Source: CAD feature listing. Evaluate the final solid. Frame: model axes, mm. Face numbers are marked on the shaded views. A direction names the side the tool comes from. Give positions to 0.01 mm unless a question says otherwise; leave off trailing zeros. Write each loop counter-clockwise with the first axis right and the second up, starting at its lowest first coordinate (ties: lowest second). Pieces come first, ordered by that corner, then holes. Notation, with made-up numbers: M 21,8 L 30,8 A17 cw 30,21 Z; hole C -1.75,9.25 d5. An arc over 180 degrees is marked long. Use CSV: the item, a comma, the result in double quotes. Start each with the question number.
Autodesk Inventor part; units mm, degrees
ref_plane "YZ Plane" through (0, 0, 0) normal (1, 0, 0) x (0, 1, 0)
ref_plane "XZ Plane" through (0, 0, 0) normal (0, 1, 0) x (-1, 0, 0)
ref_plane "XY Plane" through (0, 0, 0) normal (0, 0, 1) x (1, 0, 0)
sketch "スケッチ1" plane through (0, 0, 0) normal (0, 0, 1) x (1, 0, 0)
  line L0 (-12.5, 3.2) -> (-11.75, 0)
  line L1 (-11.75, 0) -> (11.75, 0)
  line L2 (11.75, 0) -> (12.5, 3.2)
  line L3 (12.5, 3.2) -> (19.5, 3.2)
  line L4 (19.5, 3.2) -> (19.5, -4)
  line L5 (19.5, -4) -> (-19.5, -4)
  line L6 (-19.5, -4) -> (-19.5, 3.2)
  line L7 (-19.5, 3.2) -> (-12.5, 3.2)
  circle A0 centre (0, -21) radius 12.7 construction
  line L8 (-5.5, -4) -> (5.5, -4) construction
  line L9 (5.5, -4) -> (5.5, -7.5) construction
  line L10 (5.5, -7.5) -> (-5.5, -7.5) construction
  line L11 (-5.5, -7.5) -> (-5.5, -4) construction
  circle A1 centre (0, -21) radius 14.7 construction
  line L12 (-19.5, -21) -> (19.5, -21) construction
  line L13 (-18.75, -24.8) -> (-13.25, -24.8) construction
  line L14 (-13.25, -24.8) -> (-13.25, -27.8) construction
  line L15 (-13.25, -27.8) -> (-18.75, -27.8) construction
  line L16 (-18.75, -27.8) -> (-18.75, -24.8) construction
  line L17 (-16, -27.8) -> (-16, -14.8) construction
  line L18 (-18.75, -14.8) -> (-13.25, -14.8) construction
  line L19 (-13.25, -14.8) -> (-13.25, -17.2) construction
  line L20 (-13.25, -17.2) -> (-18.75, -17.2) construction
  line L21 (-18.75, -17.2) -> (-18.75, -14.8) construction
  line L22 (-14.5, -14.8) -> (-14.5, -27.8) construction
  line L23 (-17.5, -14.8) -> (-17.5, -27.8) construction
  point P0 (0, 0)
  point P1 (0, 0)
  point P2 (0, -4)
  dimension "d0" = 4
  dimension "d1" = 3.2
  dimension "d2" = 23.5
  dimension "d3" = 25
  dimension "d4" = 39
  dimension "d5" = 25.4
  dimension "d6" = 3.5
  dimension "d7" = 21
  dimension "d8" = 11
  dimension "d9" = 2
  dimension "d11" = 5.5
  dimension "d12" = 3
  dimension "d13" = 5.5
  dimension "d14" = 2.4
  dimension "d15" = 10
  dimension "d16" = 1.5
  dimension "d17" = 1.5
  dimension "d18" = 3.8
  dimension "d19" = 16
extrude "押し出し1" add sketch "スケッチ1" along normal blind 46
sketch "スケッチ2" plane through (0, 0, 0) normal (0, 0, -1) x (-1, 0, 0)
  line L0 (19.5, -4) -> (-19.5, -4)
  circle A0 centre (0, -21) radius 12.7
  line L1 (19.5, -21) -> (-19.5, -21)
  line L2 (-19.5, -21) -> (-19.5, -4)
  line L3 (19.5, -4) -> (19.5, -21)
  point P0 (0, 0)
  point P1 (-12.7, -21)
  point P2 (12.7, -21)
extrude "押し出し2" add sketch "スケッチ2" against normal blind 31.5 contours L3 L1 A0 L2 L0
sketch "スケッチ3" plane through (0, 0, 31.5) normal (0, 0, 1) x (1, 0, 0)
  line L0 (-19.5, -4) -> (19.5, -4)
  line L1 (-19.5, -4) -> (-19.5, -21)
  line L2 (-19.5, -21) -> (-12.7, -21)
  arc A0 (12.7, -21) -> (-12.7, -21) centre (0, -21) ccw
  line L3 (12.7, -21) -> (19.5, -21)
  line L4 (19.5, -21) -> (19.5, -4)
  circle A1 centre (0, -21) radius 15
  point P0 (0, 0)
  point P1 (-15, -21)
  point P2 (15, -21)
  dimension "d24" = 30
extrude "押し出し3" add sketch "スケッチ3" along normal up to surface (14.5 mm away) contours L0 L4 L3 A1 L2 L1
sketch "スケッチ7" plane through (-19.5, -21, 0) normal (0, -1, 0) x (1, 0, 0)
  line L0 (6.8, 0) -> (0, 0) construction
  line L1 (6.8, 0) -> (6.8, 31.5) construction
  line L2 (4.5, 31.5) -> (6.8, 31.5) construction
  line L3 (4.5, 31.5) -> (4.5, 46) construction
  line L4 (4.5, 46) -> (0, 46) construction
  line L5 (0, 0) -> (0, 46) construction
  line L6 (3.5, 0) -> (3.5, 31.5) construction
  circle A0 centre (3.5, 6) radius 2.85
  circle A1 centre (3.5, 25.5) radius 2.85
  point P0 (19.5, 0)
  dimension "d34" = 16
  dimension "d35" = 5.7
  dimension "d36" = 6
  dimension "d37" = 6
extrude "押し出し6" cut sketch "スケッチ7" against normal through all
sketch "スケッチ9" plane through (-19.5, -21, 0) normal (0, -1, 0) x (1, 0, 0)
  circle A0 centre (3.5, 25.5) radius 2.85
  circle A1 centre (3.5, 6) radius 2.85
  circle A2 centre (3.5, 25.5) radius 1.6
  circle A3 centre (3.5, 6) radius 1.6
  point P0 (19.5, 0)
  dimension "d43" = 3.2
extrude "押し出し8" add sketch "スケッチ9" against normal blind 3.8
mirror "ミラー2" about plane through (0, 0, 0) normal (1, 0, 0) of "押し出し6", "押し出し8"
sketch "スケッチ10" plane through (0, 0, 0) normal (0, 0, -1) x (-1, 0, 0)
  circle A0 centre (0, -21) radius 14.7
  line L0 (-19.5, -21) -> (-12.7, -21)
  line L1 (12.7, -21) -> (19.5, -21)
  line L2 (-19.5, 3.2) -> (-19.5, -21)
  line L3 (19.5, 3.2) -> (19.5, -21)
  line L4 (-19.5, -14) -> (-6.3166, -7.7263)
  line L5 (6.3166, -7.7263) -> (19.5, -14)
  arc A1 (12.7, -21) -> (-12.7, -21) centre (0, -21) ccw
  line L6 (-19.5, 3.2) -> (-12.5, 3.2)
  line L7 (-12.5, 3.2) -> (-11.75, 0)
  line L8 (-11.75, 0) -> (11.75, 0)
  line L9 (11.75, 0) -> (12.5, 3.2)
  line L10 (12.5, 3.2) -> (19.5, 3.2)
  point P0 (0, 0)
  dimension "d46" = 7
extrude "押し出し9" cut sketch "スケッチ10" against normal through all contours A0 L4 L2 L6 L7 L8 L9 L10 L3 L5
sketch "スケッチ11" plane through (-19.5, -21, 0) normal (0, -1, 0) x (1, 0, 0)
  line L0 (-33.1912, 72.2952) -> (57.3732, 72.2952)
  line L1 (57.3732, 72.2952) -> (57.3732, -15.6553)
  line L2 (57.3732, -15.6553) -> (-33.1912, -15.6553)
  line L3 (-33.1912, -15.6553) -> (-33.1912, 72.2952)
  point P0 (19.5, 0)
extrude "押し出し10" cut sketch "スケッチ11" against normal blind 0.2
fillet "フィレット1" radius 1 2 edges at (-9.012, -9.009, 38.75) (9.012, -9.009, 38.75)
equation "\"d17\" = d16"
equation "\"d44\" = d18"
properties part number "led_holder_02"
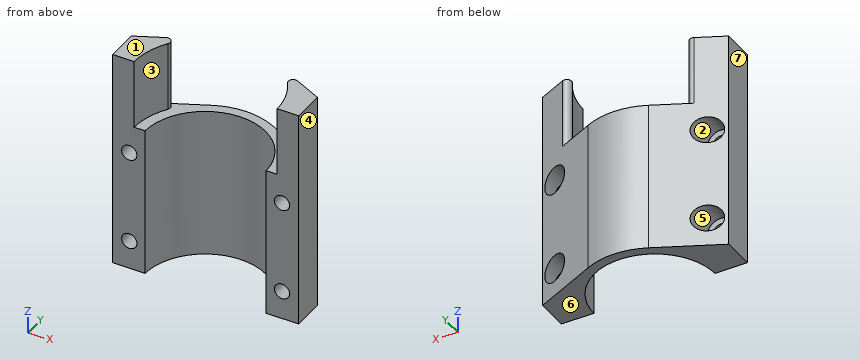
1. Section C-C on z = 32. Return loops of the section in (x, y).
2. Section A-A on y = -16.25. Return loops of the section in (x, z), then the cut area to 3 significant figures.
3. Line query: probe 1 along Z at (x, y) = (-16, -13.5); probe 2 along Z at (x, y) = (16, -18.8); probe 3 along X at (y, z) = (-16.75, 24.5). Output: solid intervals per line, ascending.
4. Pull-direction query (X, two-part tool) for the marked faces 4, 5, 6 and 7; classes: released by +X, released by -X, zero draft, split by the parting line, or undercut.
5. First-contact query: pin 1 (4.5 mm diameter, centred on x = -15, z = 27, fed in from +Y); pin 2 (4 mm diameter, centred on x = -16, z = 6, fed in from -Y); pin 3 (5 mm diameter, centred on x = -16, z = 25.5, fed in from +Y); pin 4 (4.5 mm diameter, centred on x = 14.5, z = 26, fed in from +Y). Flat tips, straight axial feed; report the tip coordinate or a pass-through.
6. Access query for the marked faces 1, 2 and 3. Directions: +Z, -Z, +X, -X, +Y, -Y. A direction counts if a zero-diameter tool reaches every point of the face in a straight line with its end or side. Return the directions, or none.
7. Section B-B on x = -16. Return loops of the section in (y, z).
8. Section D-D on y = -9.5. Return loops of the section in (x, z), then the cut area to 3 significant figures.
Resolved:
1,outline,"M -19.5,-20.8 L -15,-20.8 A15 cw -12.52,-12.73 A1 ccw -13.78,-11.28 L -19.5,-14 Z; M 12.52,-12.73 A15 cw 15,-20.8 L 19.5,-20.8 L 19.5,-14 L 13.78,-11.28 A1 ccw Z"
2,outline,"M -19.5,0 L -11.78,0 L -11.78,31.5 L -14.23,31.5 L -14.23,46 L -19.5,46 Z; M 11.78,0 L 19.5,0 L 19.5,46 L 14.23,46 L 14.23,31.5 L 11.78,31.5 Z; hole C -16,6 d5.7; hole C -16,25.5 d5.7; hole C 16,6 d5.7; hole C 16,25.5 d5.7"
2,area,"537 mm2"
3,probe 1,"z = 0 to 3.15, 8.85 to 22.65, 28.35 to 46"
3,probe 2,"z = 0 to 4.4, 7.6 to 23.9, 27.1 to 46"
3,probe 3,"x = -19.5 to -18.67, -13.33 to -11.97, 11.97 to 13.33, 18.67 to 19.5"
4,face 4,"released by +X"
4,face 5,"undercut"
4,face 6,"zero draft"
4,face 7,"released by -X"
5,pin 1,"stops at y = -10.79"
5,pin 2,"stops at y = -20.8"
5,pin 3,"stops at y = -17.2"
5,pin 4,"stops at y = -10.55"
6,face 1,"+Z, +X, -X, +Y, -Y"
6,face 2,"+Y"
6,face 3,"+Z, -Y"
7,outline,"M -20.8,0 L -12.33,0 L -12.33,3.15 L -17.2,3.15 L -17.2,4.4 L -20.8,4.4 Z; M -20.8,7.6 L -17.2,7.6 L -17.2,8.85 L -12.33,8.85 L -12.33,22.65 L -17.2,22.65 L -17.2,23.9 L -20.8,23.9 Z; M -20.8,27.1 L -17.2,27.1 L -17.2,28.35 L -12.33,28.35 L -12.33,46 L -20.8,46 Z"
8,outline,"M -10.04,0 L -5.39,0 L -5.39,31.5 L -10.04,31.5 Z; M 5.39,0 L 10.04,0 L 10.04,31.5 L 5.39,31.5 Z"
8,area,"293 mm2"
